```python
from build123d import *

# Parameters (mm, degrees)
F0_W     = 30
F0_H     = 60
F0_R     = 1.625
F1_DEPTH = 5
F2_W     = 5
F2_H     = 25
F3_DEPTH = 30
F4_R     = 1.625
F5_DEPTH = 25
F6_R     = 1.625
F7_DEPTH = 3
F8_R     = 4.99999


# Not quite as in the source:
# - a fillet or chamfer is up to 0.001 mm smaller than in the source, because OpenCascade refuses the exact size


with BuildPart() as f1:
    # F0 (on Top) → F1 (new body)
    with BuildSketch(Plane.XY):
        Rectangle(F0_W, F0_H)
        with Locations((0, 7.5)):
            Circle(F0_R, mode=Mode.SUBTRACT)
        with Locations((0, 22.5)):
            Circle(F0_R, mode=Mode.SUBTRACT)
    extrude(amount=F1_DEPTH)

    # F2 (on face) → F3 (join)
    with BuildSketch(Plane.YZ.offset(15)):
        with Locations((-27.5, 17.5)):
            Rectangle(F2_W, F2_H)
    extrude(amount=-F3_DEPTH)

    # F4 (on face) → F5 (cut)
    with BuildSketch(Plane(origin=(0, -25, 0), x_dir=(-1, 0, 0), z_dir=(0, 1, 0))):
        with Locations((0, 17.5)):
            Circle(F4_R)
    extrude(amount=-F5_DEPTH, mode=Mode.SUBTRACT)

    # F6 (on face) → F7 (cut)
    with BuildSketch(Plane(origin=(0, -25, 0), x_dir=(-1, 0, 0), z_dir=(0, 1, 0))):
        Polygon((3.5, 15.4792740578), (3.5, 19.5207259422), (0, 21.5414518843), (-3.5, 19.5207259422), (-3.5, 15.4792740578), (0, 13.4585481157), align=None)
        with Locations((0, 17.5)):
            Circle(F6_R, mode=Mode.SUBTRACT)
    extrude(amount=-F7_DEPTH, mode=Mode.SUBTRACT)

    # F8 (radius 5 in the source; OpenCascade refuses exactly that, so slightly less here)
    f8_edges = [f1.edges().sort_by_distance(p)[0] for p in [
        (0, 30, 5),
        (15, 30, 2.5),
        (-15, 30, 2.5),
        (15, 2.5, 5),
        (-15, 2.5, 5),
        (-15, -25, 17.5),
        (0, -25, 30),
        (15, -25, 17.5),
        (-15, -27.5, 30),
        (15, -27.5, 30),
    ]]
    fillet(f8_edges, radius=F8_R)


solid = f1.part
```
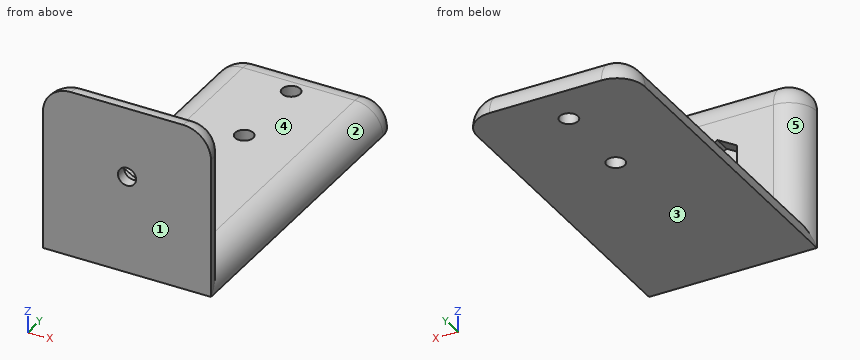
Read the model definition and answer for the solid it produces. Units are mm, in the model's axes. Face numbers are marked on the shaded views. A direction names the side the tool comes from. Round coordinates to 2 decimals unless told otherwise and drop trailing zeros. One line per item, written item: value.
Q1. Which of the six approach directions +Z, -Z, +X, -X, +Y, -Y give full straight-line access (tool end or side, diameter ignored) to the marked faces 1, 2, 3, 4 and 5?
Data:
face 1: +Z, -Z, +X, -X, -Y
face 2: +Z, +X, +Y
face 3: -Z, +X, -X, +Y, -Y
face 4: +Z, +X, -X, +Y
face 5: +Z, -X, +Y
Q2. Find section D-D on z = 3. Count the separate pieces of the cut face and the enclosed holes in it, plus the area to 3 significant figures.
Data:
separate pieces: 1
enclosed holes: 2
area: 1,630 mm2
Q3. Flat-ended cylindrical pins translate along their axes: pin 1 Ø2 at (x, z) = (-0.5, 16) entering from +Y; pin 2 Ø10 at (y, z) = (-21, 13.5) entering from -X; pin 3 Ø4 at (x, z) = (-3, 19.5) entering from +Y. Find the tip coordinate at first contact, or state that the pin passes through.
Data:
pin 1: y = -28
pin 2: x = -13
pin 3: y = -25
Q4. Straight lines are drawn through the part: line 1 (Y direction, x = 0, z = 3.1) (3 decimals); line 2 (Y direction, x = 0.25, z = 4); line 3 (Z direction, x = -3.75, y = -14.5). For each, find the intervals that lie inside material, in ascending order. Write a range as [from, to].
Data:
line 1: [-30, 5.875], [9.125, 20.875], [24.125, 28.923]
line 2: [-30, 5.89], [9.11, 20.89], [24.11, 28]
line 3: [0, 5]
